Work out the finished part from the listing and answer in its coordinate system (mm). Face numbers are marked on the shaded views. Coordinates: 2 decimals unless noted, no trailing zeros. Write each loop counter-clockwise with the first axis right and the second up, starting at its lowest first coordinate (ties: lowest second). Pieces come first, ordered by that corner, then holes. Notation, with made-up numbers: M -22.75,74 L 31.25,74 A15 ccw 31.25,82 Z; hole C 44,31.25 d1. An arc over 180 degrees is marked long. Answer as CSV lines item,"result". Start each with the question number.
(1) A cutting plane is placed at A-A on y = -13. Give the vertices of the cut face in (x, z).
(2) Find the intervals of material crossed by L1, parallel to Z at x = 99, y = -20; L2, parallel to Z at x = 90, y = -21; L3, parallel to X at y = -21, z = -74.5, in increasing order. Write a range as [from, to].
(3) A cutting plane is placed at B-B on y = -20. Give the vertices of the cut face in (x, z), then the cut area to 3 significant figures.
(4) A cutting plane is placed at D-D on x = 25.5. Give the vertices of the cut face in (y, z), then the cut area to 3 significant figures.
(5) A cutting plane is placed at C-C on z = -10.5. Give the vertices of the cut face in (x, y), then the cut area to 3 significant figures.
(6) Flat-ended cylindrical pins translate along their axes: P1, Ø12, axis at y = -21, z = -75.5, coming from the +X side; P2, Ø1, axis at y = -27.5, z = -54, coming from the +X side. Find the tip coordinate at first contact, or state that the pin passes through.
(7) The mould has two halves that part along Y. Classify the marked faces 1, 2 and 3: released by +Y, released by -Y, zero draft, split by the parting line, or undercut.
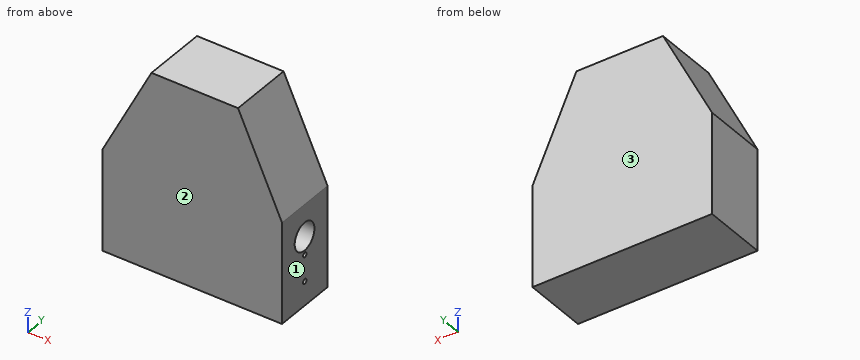
from build123d import *

# Parameters (mm, degrees)
F1_DEPTH = 40
F2_R     = 1.5
F3_DEPTH = 25
F4_R     = 8.674153
F5_DEPTH = 25


with BuildPart() as f1:
    # F0 (on Front) → F1 (new body)
    with BuildSketch(Plane.XZ):
        Polygon((76.767643, 2.10375), (27.992256, 2.10375), (-2.5816, -57.89625), (-2.5816, -120.89625), (109.4184, -120.89625), (109.4184, -59.39625), (109.4184, -57.89625), (81.992256, 2.10375), align=None)
    extrude(amount=F1_DEPTH)

    # F2 (on face) → F3 (cut)
    with BuildSketch(Plane.YZ.offset(109.4184)):
        with Locations((-20, -105.89625)):
            Circle(F2_R)
        with Locations((-20, -89.39625)):
            Circle(F2_R)
    extrude(amount=-F3_DEPTH, mode=Mode.SUBTRACT)

    # F4 (on face) → F5 (cut)
    with BuildSketch(Plane.YZ.offset(109.4184)):
        with Locations((-20.189999, -77.86797)):
            Circle(F4_R)
    extrude(amount=-F5_DEPTH, mode=Mode.SUBTRACT)


solid = f1.part
Here are the results:
1,outline,"M -2.58,-120.9 L 109.42,-120.9 L 109.42,-82.72 L 84.42,-82.72 L 84.42,-73.02 L 109.42,-73.02 L 109.42,-57.9 L 81.99,2.1 L 27.99,2.1 L -2.58,-57.9 Z"
2,L1,"z = [-120.9, -107.4], [-104.4, -90.9], [-87.9, -86.54], [-69.2, -35.1]"
2,L2,"z = [-120.9, -107.01], [-104.78, -90.51], [-88.28, -86.5], [-69.23, -15.41]"
2,L3,"x = [-2.58, 84.42]"
3,outline,"M -2.58,-120.9 L 109.42,-120.9 L 109.42,-107.4 L 84.42,-107.4 L 84.42,-104.4 L 109.42,-104.4 L 109.42,-90.9 L 84.42,-90.9 L 84.42,-87.9 L 109.42,-87.9 L 109.42,-86.54 L 84.42,-86.54 L 84.42,-69.2 L 109.42,-69.2 L 109.42,-57.9 L 81.99,2.1 L 27.99,2.1 L -2.58,-57.9 Z"
3,area,"11,500 mm^2"
4,outline,"M -40,-120.9 L 0,-120.9 L 0,-2.79 L -40,-2.79 Z"
4,area,"4,720 mm^2"
5,outline,"M 21.57,-40 L 87.75,-40 L 87.75,0 L 21.57,0 Z"
5,area,"2,650 mm^2"
6,P1,"stops at x = 84.42"
6,P2,"stops at x = 107.87"
7,face 1,"zero draft"
7,face 2,"released by -Y"
7,face 3,"released by +Y"
